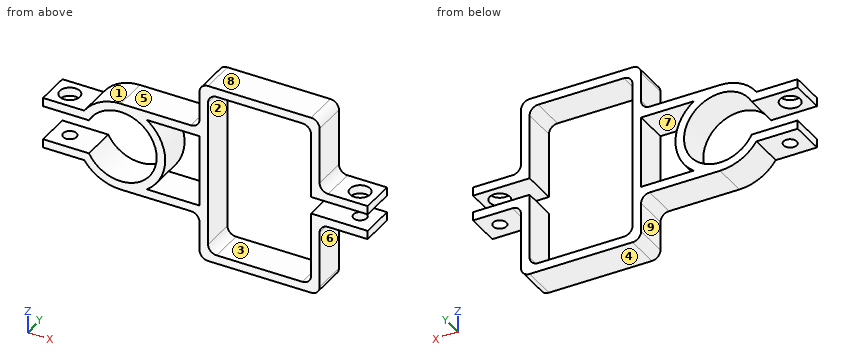
Autodesk Inventor part; units mm, degrees
ref_plane "YZ Plane" through (0, 0, 0) normal (1, 0, 0) x (0, 1, 0)
ref_plane "XZ Plane" through (0, 0, 0) normal (0, 1, 0) x (-1, 0, 0)
ref_plane "XY Plane" through (0, 0, 0) normal (0, 0, 1) x (1, 0, 0)
sketch "Sketch1" plane through (0, 0, 0) normal (0, 1, 0) x (-1, 0, 0)
  line L0 (0, 0) -> (38.1, 0)
  line L1 (38.1, 0) -> (38.1, -60.96)
  line L2 (38.1, -60.96) -> (0, -60.96)
  line L3 (-3.175, 3.175) -> (41.275, 3.175)
  line L4 (41.275, 3.175) -> (41.275, -64.135)
  line L5 (41.275, -64.135) -> (-3.175, -64.135)
  line L6 (-3.175, -36.83) -> (-20.955, -36.83)
  line L7 (-20.955, -36.83) -> (-20.955, -33.655)
  line L8 (-20.955, -33.655) -> (0, -33.655)
  line L9 (0, -33.655) -> (0, -44.417)
  line L10 (-3.175, -24.13) -> (-20.955, -24.13)
  line L11 (-20.955, -24.13) -> (-20.955, -27.305)
  line L12 (-20.955, -27.305) -> (0, -27.305)
  line L13 (0, -27.305) -> (0, -17.217)
  line L14 (0, -60.96) -> (0, -33.655)
  line L15 (0, -27.305) -> (0, 0)
  line L16 (-3.175, -24.13) -> (-3.175, 3.175)
  line L17 (-3.175, -64.135) -> (-3.175, -36.83)
  arc A0 (82.211, -24.13) -> (82.211, -36.83) centre (70.485, -30.48) ccw
  line L18 (99.2103, -36.83) -> (82.211, -36.83)
  line L19 (99.2103, -40.005) -> (99.2103, -36.83)
  line L20 (82.211, -24.13) -> (99.2103, -24.13)
  line L21 (99.2103, -24.13) -> (99.2103, -20.955)
  line L22 (99.2103, -20.955) -> (83.9703, -20.955)
  line L23 (83.9703, -40.005) -> (99.2103, -40.005)
  arc A1 (83.9703, -20.955) -> (83.9703, -40.005) centre (70.485, -30.48) ccw
  line L24 (41.275, -13.97) -> (70.485, -13.97)
  line L25 (70.485, -46.99) -> (41.275, -46.99)
  line L26 (60.7506, -17.145) -> (41.275, -17.145)
  line L27 (60.7506, -43.815) -> (41.275, -43.815)
  point P0 (41.275, -30.48)
  dimension "d0" = 38.1
  dimension "d1" = 60.96
  dimension "d2" = 3.175
  dimension "d3" = 3.175
  dimension "d4" = 3.175
  dimension "d5" = 3.175
  dimension "d6" = 3.175
  dimension "d7" = 3.175
  dimension "d8" = 3.175
  dimension "d9" = 17.78
  dimension "d10" = 6.35
  dimension "d23" = 26.67
  dimension "d25" = 3.175
  dimension "d27" = 15.24
  dimension "d28" = 6.35
  dimension "d29" = 6.35
  dimension "d30" = 3.175
  dimension "d31" = 3.175
  dimension "d32" = 12.7
  dimension "d33" = 3.175
  dimension "d34" = 3.175
extrude "Extrusion1" add sketch "Sketch1" along normal blind 12.7 contours L15 L13 L12 L11 L10 L16 L3 L4 L5 L17 L6 L7 L8 L9 L14 L2 L1 L0 | L24 A1 L26 L4 | A1 L22 L21 L20 A0 L18 L19 L23 | L27 A1 L25 L4
sketch "Sketch2" plane through (3.175, 0, -24.13) normal (0, 0, 1) x (1, 0, 0)
  circle A0 centre (11.43, 6.35) radius 2.4511
  line L0 (0, 12.7) -> (17.78, 12.7)
  line L1 (17.78, 0) -> (17.78, 12.7)
  point P0 (-3.175, 0)
  dimension "d13" = 4.9022
  dimension "d14" = 6.35
  dimension "d15" = 6.35
extrude "Extrusion2" cut sketch "Sketch2" against normal blind 23.8125
sketch "Sketch3" plane through (3.175, 0, -24.13) normal (0, 0, 1) x (1, 0, 0)
  circle A0 centre (11.43, 6.35) radius 2.4511
  circle A1 centre (11.43, 6.35) radius 3.7211
  point P0 (-3.175, 0)
  dimension "d18" = 1.27
extrude "Extrusion3" cut sketch "Sketch3" against normal blind 9.525
fillet "Fillet1" radius 3.175 4 edges at (-38.1, 6.35, -60.96) (0, 6.35, -60.96) (0, 6.35, 0) (-38.1, 6.35, 0)
fillet "Fillet2" radius 3.175 8 edges at (-41.275, 6.35, 3.175) (-41.275, 6.35, -64.135) (3.175, 6.35, -64.135) (3.175, 6.35, 3.175) (3.175, 6.35, -24.13) (3.175, 6.35, -36.83) (-41.275, 6.35, -13.97) (-41.275, 6.35, -46.99)
sketch "Sketch4" plane through (-99.2103, 0, -20.955) normal (0, 0, 1) x (1, 0, 0)
  circle A0 centre (6.35, 6.35) radius 2.4511
  line L0 (0, 12.7) -> (15.24, 12.7)
  line L1 (0, 0) -> (0, 12.7)
  point P0 (99.2103, 0)
  dimension "d35" = 4.9022
  dimension "d36" = 6.35
  dimension "d37" = 6.35
extrude "Extrusion4" cut sketch "Sketch4" against normal blind 23.8125
sketch "Sketch5" plane through (-99.2103, 0, -20.955) normal (0, 0, 1) x (1, 0, 0)
  circle A0 centre (6.35, 6.35) radius 2.4511
  circle A1 centre (6.35, 6.35) radius 3.7211
  point P0 (99.2103, 0)
  dimension "d40" = 1.27
extrude "Extrusion5" cut sketch "Sketch5" against normal blind 9.525
equation "\"d3\" = d2"
equation "\"d4\" = d2"
equation "\"d5\" = d2"
equation "\"d6\" = d2"
equation "\"d7\" = d2"
equation "\"d8\" = d2"
equation "\"d25\" = d2"
equation "\"d29\" = d28"
equation "\"d30\" = d2"
equation "\"d31\" = d2"
equation "\"d33\" = d2"
equation "\"d34\" = d2"
equation "\"d15\" = d14"
equation "\"d37\" = d36"
equation "\"d24\" = d2"
equation "\"d26\" = d2"
properties part number "kinect mount" material "PC/ABS Plastic"
Design review of the part built by this model. Coordinates are the model's own, in mm. Face numbers are marked on the shaded views. A direction names the side the tool comes from. Round coordinates to 2 decimals unless told otherwise and drop trailing zeros. Loops run counter-clockwise (first coordinate to the right, second up) from the corner with the lowest first, then second, coordinate; pieces in that order, holes last. Notation, with made-up numbers: M 69.5,24.5 L 116.5,24.5 A24 cw 116.5,55.5 Z; hole C -6.5,82.5 d7. An arc over 180 degrees is marked long. Answer as a JSON object with one key per item and string values.
Item 1: The part is to be moulded in two halves that separate along Z. For the marked faces 1, 2, 3 and 4, say which applies: pulls with the +Z half, pulls with the -Z half, needs draft (parallel to the pull), parting line crosses it, or undercut.
Answer sheet:
{"face 1": "pulls with the +Z half", "face 2": "undercut", "face 3": "undercut", "face 4": "pulls with the -Z half"}
Item 2: We need section A-A on x = -28. Give the boundary of the cut face in (y, z) (3 decimals).
Answer sheet:
{"outline": "M 0,-64.135 L 12.7,-64.135 L 12.7,-60.96 L 0,-60.96 Z; M 0,0 L 12.7,0 L 12.7,3.175 L 0,3.175 Z"}
Item 3: We need section B-B on z = -51.5. Give the boundary of the cut face in (x, y) (3 decimals).
Answer sheet:
{"outline": "M -41.275,0 L -38.1,0 L -38.1,12.7 L -41.275,12.7 Z; M 0,0 L 3.175,0 L 3.175,12.7 L 0,12.7 Z"}
Item 4: We need section D-D on y = 6.35. State how many separate pieces and enclosed holes the cut face has, and give its area (3 significant figures).
Answer sheet:
{"separate pieces": "5", "enclosed holes": "1", "area": "1,180 mm^2"}
Item 5: Machinability: for the marked faces 5, 6, 7, 8 and 9, which of the approach directions +Z, -Z, +X, -X, +Y, -Y give a long, thin tool a straight path to every point of the face, cutting with its end or side? Answer none if there is none.
Answer sheet:
{"face 5": "+Z, -X, +Y, -Y", "face 6": "-Z, +X, +Y, -Y", "face 7": "+Y, -Y", "face 8": "+Z, +X, -X, +Y, -Y", "face 9": "-Z, -X, +Y, -Y"}
Item 6: Clearance check with flat-ended pins moving along their axes: P1, Ø4, axis at y = 4.5, z = -15, coming from the -X side; P2, Ø5.5, axis at y = 5.5, z = -54.5, coming from the -X side (3 decimals); P3, Ø6.5, axis at x = -94, y = 4, coming from the -Z side (3 decimals). State where each tip first meets the part, or that it passes through.
Answer sheet:
{"P1": "stops at x = -80.02", "P2": "stops at x = -41.275", "P3": "stops at z = -40.005"}
Item 7: We need section C-C on z = -38.5. Give the boundary of the cut face in (x, y) (3 decimals), and give its area (3 significant figures).
Answer sheet:
{"outline": "M -99.21,0 L -81.139,0 L -81.139,12.7 L -99.21,12.7 Z; M -59.831,0 L -56.054,0 L -56.054,12.7 L -59.831,12.7 Z; M -41.275,0 L -38.1,0 L -38.1,12.7 L -41.275,12.7 Z; M 0,0 L 3.554,0 L 3.554,12.7 L 0,12.7 Z; hole C -92.86,6.35 d4.902", "area": "344 mm^2"}
Item 8: Wall thickness on L1, parallel to X at y = 11.5, z = -4 (3 decimals); L2, parallel to Z at x = -84.5, y = 9.5 (3 decimals); L3, parallel to Z at x = 13, y = 0.5 (3 decimals): over which ranges is each line inside the solid? List them lowest first. Write a range as from..to.
Answer sheet:
{"L1": "x = -41.275..-38.1, 0..3.175", "L2": "z = -40.005..-36.83, -24.13..-20.955", "L3": "z = -36.83..-33.655, -27.305..-24.13"}
